from build123d import *
from OCP.BRepFilletAPI import BRepFilletAPI_MakeChamfer
from build123d.topology import SkipClean

# Parameters (mm, degrees)
SKETCH1_W                  = 0.762
SKETCH1_H                  = 6.096
SKETCH2_R                  = 3.175
BOSS_EXTRUDE1_DEPTH        = 19.05
CUT_EXTRUDE1_START         = -4.445
CUT_EXTRUDE1_DEPTH         = 4.445
BOSS_EXTRUDE2_DEPTH        = 4.445
BOSS_EXTRUDE3_DEPTH        = 4.826
M6_5_CLEARANCE_HOLE1_D     = 7.45744
M6_5_CLEARANCE_HOLE1_DEPTH = 0.9652
CHAMFER1_SIZE              = 0.9017
CHAMFER1_SIZE2             = 1.561790213


with BuildPart() as part:
    # Sketch1 → Revolve1 (revolve)
    with BuildSketch(Plane(origin=(0, 0, 0), x_dir=(-1, 0, 0), z_dir=(0, 0, -1)), mode=Mode.PRIVATE) as revolve1_sk:
        with Locations((0.381, 3.048)):
            Rectangle(SKETCH1_W, SKETCH1_H)
    revolve(revolve1_sk.sketch.rotate(Axis((0, 0, 0), (-1, 0, 0)), 270), axis=Axis((0, 0, 0), (-1, 0, 0)))

    # Sketch2 → Boss-Extrude1 (add)
    with BuildSketch(Plane(origin=(0, 0, 0), x_dir=(0, 0, -1), z_dir=(1, 0, 0))):
        with Locations(Location((0, 0, 0), (0, 0, 180))):
            Circle(SKETCH2_R)
    extrude(amount=BOSS_EXTRUDE1_DEPTH)

    # Sketch3 → Cut-Extrude1 (cut)
    with BuildSketch(Plane(origin=(19.05, 0, 0), x_dir=(0, 0, -1), z_dir=(1, 0, 0)).offset(CUT_EXTRUDE1_START)):
        with BuildLine():
            Line((3.163956488, 0.264583333), (-3.163956488, 0.264583333))
            ThreePointArc((-3.163956488, 0.264583333), (0, -3.175), (3.163956488, 0.264583333))
        make_face()
    extrude(amount=CUT_EXTRUDE1_DEPTH, mode=Mode.SUBTRACT)

    # Sketch4 → Boss-Extrude2 (add)
    with SkipClean():  # the faces are left unmerged after this step: merging them gives an invalid solid
        with BuildSketch(Plane(origin=(14.605, 0, 0), x_dir=(0, 0, -1), z_dir=(1, 0, 0))):
            with BuildLine():
                Line((-3.163956488, -0.264583333), (3.163956488, -0.264583333))
                ThreePointArc((3.163956488, -0.264583333), (0, -3.175), (-3.163956488, -0.264583333))
            make_face()
        extrude(amount=BOSS_EXTRUDE2_DEPTH)

    # Sketch5 → Boss-Extrude3 (add)
    with SkipClean():  # the faces are left unmerged after this step: merging them gives an invalid solid
        with BuildSketch(Plane.ZY.offset(0.762)):
            Polygon((-5.381943739, 0), (-2.69097187, 4.6609), (2.69097187, 4.6609), (5.381943739, 0), (2.69097187, -4.6609), (-2.69097187, -4.6609), align=None)
        extrude(amount=BOSS_EXTRUDE3_DEPTH)

    # M6.5 Clearance Hole1
    with Locations(Plane.ZY.offset(5.588)):
        with Locations((0, 0)):
            Hole(M6_5_CLEARANCE_HOLE1_D / 2, depth=M6_5_CLEARANCE_HOLE1_DEPTH)

    # Chamfer1: one chamfer whose edges measure the first distance from different faces: ONE call of the kernel's chamfer builder (chamfer() names one face for all edges)
    chamfer1_edges_1 = [part.edges().sort_by_distance(p)[0] for p in [
        (19.05, -3.175, 0),
    ]]
    chamfer1_side_1 = [part.faces().sort_by_distance(p)[0] for p in [
        (19.05, -1.491577602, 0),
    ]]
    chamfer1_edges_2 = [part.edges().sort_by_distance(p)[0] for p in [
        (19.05, 3.175, 0),
    ]]
    chamfer1_side_2 = [part.faces().sort_by_distance(p)[0] for p in [
        (19.05, 1.491577602, 0),
    ]]
    chamfer1 = BRepFilletAPI_MakeChamfer(part.part.solid().wrapped)
    for e in chamfer1_edges_1:
        chamfer1.Add(CHAMFER1_SIZE, CHAMFER1_SIZE2, e.wrapped, chamfer1_side_1[0].wrapped)  # the first distance lies on this face
    for e in chamfer1_edges_2:
        chamfer1.Add(CHAMFER1_SIZE, CHAMFER1_SIZE2, e.wrapped, chamfer1_side_2[0].wrapped)  # the first distance lies on this face
    add(Compound.cast(chamfer1.Shape()), mode=Mode.REPLACE)


solid = part.part
Build history of the part. All positions in model axes, mm. A direction names the side the tool comes from. Coordinates: 2 decimals unless noted, no trailing zeros. Write each loop counter-clockwise with the first axis right and the second up, starting at its lowest first coordinate (ties: lowest second). Pieces come first, ordered by that corner, then holes.
(1) Cut at A-A on x = 16.75. List the corners of the cut face in (y, z) (3 decimals).
(2) 3-axis set-ups, long thin cutter, end or side, ignore diameter. For faces 4 (the flat face through (0, -3, -3)), 5 (the flat face through (17, -0.265, 0)), 6 (the flat face through (-3, -4.661, 0)): which of +Z, -Z, +X, -X, +Y, -Y reach the whole face in a straight line?
(3) Drill centre lines: line 1 (Y direction, x = -5.1, z = 0); line 2 (X direction, y = -0.25, z = 4.25); line 3 (X direction, y = 1, z = 1). Where is each one in solid material? Low to high.
(4) Cut at D-D on z = -4.75. List the corners of the cut face in (x, y).
(5) Pin check, flat tips, straight feed: pin 1 Ø4 at (x, z) = (-4, -1) entering from +Y; pin 2 Ø4 at (x, y) = (13.5, 1.5) entering from +Z (3 decimals); pin 3 Ø1.4 at (x, z) = (-4, -1) entering from -Y; pin 4 Ø6 at (y, z) = (-2.5, 1.5) entering from +X. Stop position of each tip, or through.
(6) Cut at B-B on z = 0. List the corners of the cut face in (x, y) (3 decimals).
(7) Mould opens along Y. For faces 1 (the cylindrical face through (-5.1, -3.64, 0.81)), 2 (the flat face through (-3, 4.661, 0)), 3 (the flat face through (-3.141, -2.298, 4.055)) say: pulls with the +Y half, pulls with the -Y half, needs draft (parallel to the pull), parting line crosses it, or undercut.
(8) Cut at C-C on y = -4. List the corners of the cut face in (x, z).
Working result:
1. outline: (-0.265, -3.164) - (-0.265, 3.164) arc R3.175 ccw to start; (0.265, -3.164) arc R3.175 ccw to (0.265, 3.164) - close
2. face 4: +X
2. face 5: +Z, -Z, +X
2. face 6: +Z, -Z, -X, -Y
3. line 1: y = -4.66 to -3.73, 3.73 to 4.66
3. line 2: x = -5.59 to 0
3. line 3: x = -4.62 to 19.05
4. outline: (-5.59, -1.09) - (-0.76, -1.09) - (-0.76, -3.82) - (0, -3.82) - (0, 3.82) - (-0.76, 3.82) - (-0.76, 1.09) - (-5.59, 1.09) - close
5. pin 1: stops at y = 4.66
5. pin 2: stops at z = 3.175
5. pin 3: stops at y = -4.66
5. pin 4: stops at x = 19.05
6. outline: (-5.588, -4.661) - (-0.762, -4.661) - (-0.762, -6.096) - (0, -6.096) - (0, -3.175) - (17.488, -3.175) - (19.05, -2.273) - (19.05, -0.265) - (14.605, -0.265) - (14.605, 0.265) - (19.05, 0.265) - (19.05, 2.273) - (17.488, 3.175) - (0, 3.175) - (0, 6.096) - (-0.762, 6.096) - (-0.762, 4.661) - (-5.588, 4.661) - (-5.588, 3.729) - (-4.623, 3.729) - (-4.623, -3.729) - (-5.588, -3.729) - close
7. face 1: undercut
7. face 2: pulls with the +Y half
7. face 3: pulls with the -Y half
8. outline: (-5.59, -3.07) - (-0.76, -3.07) - (-0.76, -4.6) - (0, -4.6) - (0, 4.6) - (-0.76, 4.6) - (-0.76, 3.07) - (-5.59, 3.07) - close
